```python
from build123d import *

# Parameters (mm, degrees)
BOSS_EXTRUDE1_DEPTH = 1
BOSS_EXTRUDE2_DEPTH = 10


with BuildPart() as part:
    # Sketch1 → Boss-Extrude1 (new body)
    with BuildSketch(Plane(origin=(0, 125.994845224, 0), x_dir=(0.999996103, 0, 0.002791708), z_dir=(0, -1, 0))):
        with BuildLine():
            Line((-0.618086487, 4.765287934), (-0.561019037, 5.471312241))
            ThreePointArc((-0.561019037, 5.471312241), (-5.482120778, 0.443115979), (-1.432479428, -5.310179158))
            Line((-1.432479428, -5.310179158), (-1.375411978, -4.604154851))
            Line((-1.375411978, -4.604154851), (0.618086487, -4.765287934))
            Line((0.618086487, -4.765287934), (0.561019037, -5.471312241))
            ThreePointArc((0.561019037, -5.471312241), (4.082621995, -3.685403322), (5.5, 0))
            ThreePointArc((5.5, 0), (4.36627054, 3.344500198), (1.432479428, 5.310179158))
            Line((1.432479428, 5.310179158), (1.375411978, 4.604154851))
            Line((1.375411978, 4.604154851), (-0.618086487, 4.765287934))
        make_face()
        with BuildLine():
            Line((1.376787234, -2.757386609), (-1.801775741, -2.500465592))
            ThreePointArc((-1.801775741, -2.500465592), (-2.347797606, -1.996639778), (-2.757386609, -1.376787234))
            Line((-2.757386609, -1.376787234), (-2.628926101, 0.212494254))
            Line((-2.628926101, 0.212494254), (-2.500465592, 1.801775741))
            ThreePointArc((-2.500465592, 1.801775741), (-1.996639778, 2.347797606), (-1.376787234, 2.757386609))
            Line((-1.376787234, 2.757386609), (1.801775741, 2.500465592))
            ThreePointArc((1.801775741, 2.500465592), (2.347797606, 1.996639778), (2.757386609, 1.376787234))
            Line((2.757386609, 1.376787234), (2.628926101, -0.212494254))
            Line((2.628926101, -0.212494254), (2.500465592, -1.801775741))
            ThreePointArc((2.500465592, -1.801775741), (1.996639778, -2.347797606), (1.376787234, -2.757386609))
        make_face(mode=Mode.SUBTRACT)
        with BuildLine():
            Line((-2.628926101, 0.212494254), (-2.757386609, -1.376787234))
            ThreePointArc((-2.757386609, -1.376787234), (-2.347797606, -1.996639778), (-1.801775741, -2.500465592))
            Line((-1.801775741, -2.500465592), (1.376787234, -2.757386609))
            ThreePointArc((1.376787234, -2.757386609), (1.996639778, -2.347797606), (2.500465592, -1.801775741))
            Line((2.500465592, -1.801775741), (2.628926101, -0.212494254))
            Line((2.628926101, -0.212494254), (2.757386609, 1.376787234))
            ThreePointArc((2.757386609, 1.376787234), (2.347797606, 1.996639778), (1.801775741, 2.500465592))
            Line((1.801775741, 2.500465592), (-1.376787234, 2.757386609))
            ThreePointArc((-1.376787234, 2.757386609), (-1.996639778, 2.347797606), (-2.500465592, 1.801775741))
            Line((-2.500465592, 1.801775741), (-2.628926101, 0.212494254))
        make_face()
        with BuildLine():
            ThreePointArc((1.149706447, -1.735770459), (1.348800784, -1.586020316), (1.528583278, -1.413561871))
            Line((1.528583278, -1.413561871), (1.632176868, -0.131927712))
            Line((1.632176868, -0.131927712), (1.735770459, 1.149706447))
            ThreePointArc((1.735770459, 1.149706447), (1.586020316, 1.348800784), (1.413561871, 1.528583278))
            Line((1.413561871, 1.528583278), (-1.149706447, 1.735770459))
            ThreePointArc((-1.149706447, 1.735770459), (-1.348800784, 1.586020316), (-1.528583278, 1.413561871))
            Line((-1.528583278, 1.413561871), (-1.632176868, 0.131927712))
            Line((-1.632176868, 0.131927712), (-1.735770459, -1.149706447))
            ThreePointArc((-1.735770459, -1.149706447), (-1.586020316, -1.348800784), (-1.413561871, -1.528583278))
            Line((-1.413561871, -1.528583278), (1.149706447, -1.735770459))
        make_face(mode=Mode.SUBTRACT)
        with BuildLine():
            Line((-1.413561871, -1.528583278), (1.149706447, -1.735770459))
            ThreePointArc((1.149706447, -1.735770459), (1.348800784, -1.586020316), (1.528583278, -1.413561871))
            Line((1.528583278, -1.413561871), (1.632176868, -0.131927712))
            Line((1.632176868, -0.131927712), (1.735770459, 1.149706447))
            ThreePointArc((1.735770459, 1.149706447), (1.586020316, 1.348800784), (1.413561871, 1.528583278))
            Line((1.413561871, 1.528583278), (-1.149706447, 1.735770459))
            ThreePointArc((-1.149706447, 1.735770459), (-1.348800784, 1.586020316), (-1.528583278, 1.413561871))
            Line((-1.528583278, 1.413561871), (-1.632176868, 0.131927712))
            Line((-1.632176868, 0.131927712), (-1.735770459, -1.149706447))
            ThreePointArc((-1.735770459, -1.149706447), (-1.586020316, -1.348800784), (-1.413561871, -1.528583278))
        make_face()
        with BuildLine():
            ThreePointArc((1.241016617, -0.100310503), (0.100310503, 1.241016617), (-1.241016617, 0.100310503))
            ThreePointArc((-1.241016617, 0.100310503), (-0.100310503, -1.241016617), (1.241016617, -0.100310503))
        make_face(mode=Mode.SUBTRACT)
        with BuildLine():
            ThreePointArc((-1.241016617, 0.100310503), (-0.100310503, -1.241016617), (1.241016617, -0.100310503))
            ThreePointArc((1.241016617, -0.100310503), (0.100310503, 1.241016617), (-1.241016617, 0.100310503))
        make_face()
    extrude(amount=BOSS_EXTRUDE1_DEPTH)

    # Sketch1_4 → Boss-Extrude2 (add)
    with BuildSketch(Plane(origin=(0, 125.994845224, 0), x_dir=(0.999996103, 0, 0.002791708), z_dir=(0, -1, 0))):
        with BuildLine():
            Line((-2.628926101, 0.212494254), (-2.757386609, -1.376787234))
            ThreePointArc((-2.757386609, -1.376787234), (-2.347797606, -1.996639778), (-1.801775741, -2.500465592))
            Line((-1.801775741, -2.500465592), (1.376787234, -2.757386609))
            ThreePointArc((1.376787234, -2.757386609), (1.996639778, -2.347797606), (2.500465592, -1.801775741))
            Line((2.500465592, -1.801775741), (2.628926101, -0.212494254))
            Line((2.628926101, -0.212494254), (2.757386609, 1.376787234))
            ThreePointArc((2.757386609, 1.376787234), (2.347797606, 1.996639778), (1.801775741, 2.500465592))
            Line((1.801775741, 2.500465592), (-1.376787234, 2.757386609))
            ThreePointArc((-1.376787234, 2.757386609), (-1.996639778, 2.347797606), (-2.500465592, 1.801775741))
            Line((-2.500465592, 1.801775741), (-2.628926101, 0.212494254))
        make_face()
        with BuildLine():
            ThreePointArc((1.149706447, -1.735770459), (1.348800784, -1.586020316), (1.528583278, -1.413561871))
            Line((1.528583278, -1.413561871), (1.632176868, -0.131927712))
            Line((1.632176868, -0.131927712), (1.735770459, 1.149706447))
            ThreePointArc((1.735770459, 1.149706447), (1.586020316, 1.348800784), (1.413561871, 1.528583278))
            Line((1.413561871, 1.528583278), (-1.149706447, 1.735770459))
            ThreePointArc((-1.149706447, 1.735770459), (-1.348800784, 1.586020316), (-1.528583278, 1.413561871))
            Line((-1.528583278, 1.413561871), (-1.632176868, 0.131927712))
            Line((-1.632176868, 0.131927712), (-1.735770459, -1.149706447))
            ThreePointArc((-1.735770459, -1.149706447), (-1.586020316, -1.348800784), (-1.413561871, -1.528583278))
            Line((-1.413561871, -1.528583278), (1.149706447, -1.735770459))
        make_face(mode=Mode.SUBTRACT)
    extrude(amount=-BOSS_EXTRUDE2_DEPTH)


solid = part.part
```
Read the model definition and answer for the solid it produces. Units are mm, in the model's axes. A direction names the side the tool comes from. Coordinates: 2 decimals unless noted, no trailing zeros. Write each loop counter-clockwise with the first axis right and the second up, starting at its lowest first coordinate (ties: lowest second). Pieces come first, ordered by that corner, then holes. Notation, with made-up numbers: (-10.5, -19) - (23.5, -19) arc R12 ccw to (23.5, -4) - close; hole circle Ø3 at (-32, 46). An arc over 180 degrees is marked (long way). Answer as a JSON object with one key per item and string values. Group by question number.
1. The mould has two halves that part along Z. Classify faces 5 (the flat face through (0.15, 130.92, 1.63)), 6 (the flat face through (0, 135.995, -2)), 7 (the cylindrical face through (-2.349, 130.925, -1.995)), 8 (the flat face through (0.227, 130.925, 2.628)): +Z half, -Z half, draft (parallel to the pull), parting line (faces both ways), or undercut.
2. A cutting plane is placed at B-B (x = 1). Determine the outline of the cut face in (y, z), plus the area to 3 significant figures.
3. Consider L1, parallel to Y at x = 1, z = -3.75; L2, parallel to Z at x = 1.5, y = 130.5; L3, parallel to X at y = 133.5, z = -0.75. Determine where each line is inside the solid, lowest interval first. Write a range as [from, to].
4. Each of these flat-tipped pins is pushed along its axis until it touches: P1, Ø4, axis at x = -3, y = 134.5, coming from the +Z side; P2, Ø1.5, axis at y = 131, z = 4, coming from the +X side; P3, Ø1.5, axis at x = 0.5, y = 131, coming from the -Z side; P4, Ø1, axis at x = -0.5, y = 127, coming from the -Z side. Where does it stop, or does it pass through?
5. Which of the six approach directions +Z, -Z, +X, -X, +Y, -Y give full straight-line access (tool end or side, diameter ignored) to faces 1 (the cylindrical face through (-1.995, 130.925, 2.349)), 2 (the cylindrical face through (2.349, 130.925, 1.995)), 3 (the cylindrical face through (1.995, 130.925, -2.349)), 4 (the flat face through (2.4, 125.995, -2.3))?
6. A cutting plane is placed at C-C (z = 0.75). Determine the outline of the cut face in (x, y), plus the area to 3 significant figures.
7. A cutting plane is placed at D-D (z = -2.25). Determine the outline of the cut face in (x, y).
8. A cutting plane is placed at A-A (y = 131.5). Determine the outline of the cut face in (x, z).
Worked out:
{
 "1": {"face 5": "undercut", "face 6": "draft", "face 7": "-Z half", "face 8": "+Z half"},
 "2": {"outline": "(124.99, -5.41) - (125.99, -5.41) - (125.99, -2.72) - (135.99, -2.72) - (135.99, -1.72) - (125.99, -1.72) - (125.99, 1.56) - (135.99, 1.56) - (135.99, 2.57) - (125.99, 2.57) - (125.99, 4.64) - (124.99, 4.64) - close", "area": "30.1 mm²"},
 "3": {"L1": "y = [124.99, 125.99]", "L2": "z = [-2.69, -1.44], [1.44, 2.53]", "L3": "x = [-2.7, -1.7], [1.58, 2.59]"},
 "4": {"P1": "stops at z = 2.75", "P2": "passes through", "P3": "stops at z = -2.74", "P4": "stops at z = -2.65"},
 "5": {"face 1": "+Z, -X, +Y", "face 2": "+Z, +X, +Y", "face 3": "-Z, +X, +Y", "face 4": "+Y"},
 "6": {"outline": "(-5.45, 124.99) - (5.45, 124.99) - (5.45, 125.99) - (2.7, 125.99) - (2.7, 135.99) - (1.7, 135.99) - (1.7, 125.99) - (-1.58, 125.99) - (-1.58, 135.99) - (-2.59, 135.99) - (-2.59, 125.99) - (-5.45, 125.99) - close", "area": "31.0 mm²"},
 "7": {"outline": "(-5.02, 124.99) - (5.02, 124.99) - (5.02, 125.99) - (2.11, 125.99) - (2.11, 135.99) - (-2.11, 135.99) - (-2.11, 125.99) - (-5.02, 125.99) - close"},
 "8": {"outline": "(-2.75, -1.38) arc R3.08 ccw to (-1.79, -2.51) - (1.38, -2.75) arc R3.08 ccw to (2.51, -1.79) - (2.75, 1.38) arc R3.08 ccw to (1.79, 2.51) - (-1.38, 2.75) arc R3.08 ccw to (-2.51, 1.79) - close; hole (-1.73, -1.15) arc R2.08 ccw to (-1.41, -1.53) - (1.15, -1.73) arc R2.08 ccw to (1.53, -1.41) - (1.73, 1.15) arc R2.08 ccw to (1.41, 1.53) - (-1.15, 1.73) arc R2.08 ccw to (-1.53, 1.41) - close"}
}
